Geometry check sheet. Reference: the model listing, model coordinates, mm. Face numbers are marked on the shaded views. Coordinates: 2 decimals unless noted, no trailing zeros. Write each loop counter-clockwise with the first axis right and the second up, starting at its lowest first coordinate (ties: lowest second). Pieces come first, ordered by that corner, then holes. Notation, with made-up numbers: (-10.75, -16.5) -> (4.25, -16.5) arc R27 cw to (4.25, 2.5) -> close; hole circle Ø3 at (4, 9.25). An arc over 180 degrees is marked (long way). Answer in a Markdown table with one row per item. Add a question column.
1. Mould release check, pull along Z, two halves, no side actions. Record for the marked faces 1, 2, 3 and 4: pulls with the +Z half, pulls with the -Z half, needs draft (parallel to the pull), parting line crosses it, or undercut.
2. Scan lines: L1, parallel to Z at x = 1303.5, y = 13.5; L2, parallel to Z at x = 1605, y = 19; L3, parallel to X at y = 12, z = -637. Record each from-to range of solid material in increasing order. Write a range as from..to.
3. Cross-section at B-B on x = 790. Record the cut outline in (y, z).
4. Depth check by flat-ended pin: P1, Ø1, axis at y = 34.5, z = -697.5, coming from the +X side. Enter the tip coordinate at first touch or a pass-through.
5. Cross-section at A-A on z = -89. Record the cut outline in (x, y).
6. Cross-section at C-C on y = 68. Record the cut outline in (x, z).
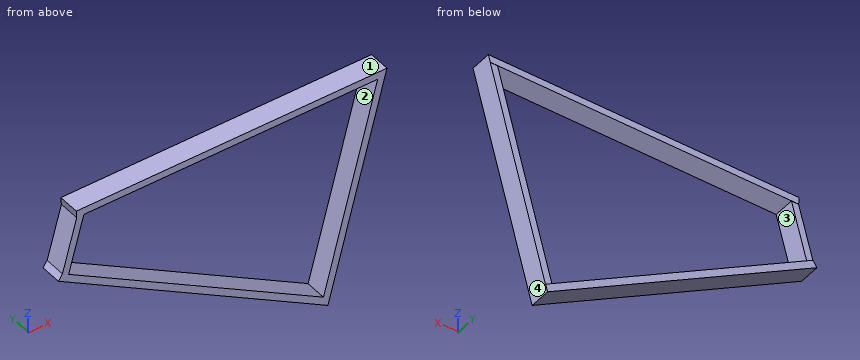
Autodesk Inventor part; units mm, degrees
ref_plane "YZ Plane" through (0, 0, 0) normal (1, 0, 0) x (0, 1, 0)
ref_plane "XZ Plane" through (0, 0, 0) normal (0, 1, 0) x (-1, 0, 0)
ref_plane "XY Plane" through (0, 0, 0) normal (0, 0, 1) x (1, 0, 0)
sketch "Sketch1" plane through (0, 0, 0) normal (0, 1, 0) x (-1, 0, 0)
  line L0 (0, 0) -> (-3000, 0) construction
  line L1 (0, 0) -> (-2598.0762, -1500) construction
  line L2 (0, 0) -> (3000, 0) construction
  arc A0 (-497.4937, 50) -> (-402.0602, -297.2332) centre (0, 0) ccw
  line L3 (-497.4937, 50) -> (-2157.4937, 50)
  line L4 (-2157.4937, 50) -> (-1841.7345, -1128.4295)
  line L5 (-2157.4937, 50) -> (-937.4937, 50) construction
  line L6 (-1841.7345, -1128.4295) -> (1158.2655, -1128.4295) construction
  line L7 (-1841.7345, -1128.4295) -> (-402.0602, -297.2332)
  arc A1 (-537.8662, 12) -> (-456.459, -284.7617) centre (0, 0) ccw
  line L8 (-2107.9712, 12) -> (-537.8662, 12)
  line L9 (-456.459, -284.7617) -> (-1817.8467, -1070.7593)
  line L10 (-2107.9712, 12) -> (-1817.8467, -1070.7593)
  dimension "d1" = 3000
  dimension "d2" = 150
  dimension "d3" = 1000
  dimension "d11" = 50
  dimension "d12" = 1660
  dimension "d13" = 1220
  dimension "d14" = 75
extrude "Extrusion2" add sketch "Sketch1" along normal blind 114
sketch "Sketch2" plane through (0, 114, 0) normal (0, 1, 0) x (1, 0, 0)
  line L0 (497.4937, -50) -> (2157.4937, -50)
  line L1 (1841.7345, 1128.4295) -> (402.0602, 297.2332)
  arc A0 (497.4937, -50) -> (402.0602, 297.2332) centre (0, 0) ccw
  line L2 (456.459, 284.7617) -> (537.8662, -12)
  line L3 (456.459, 284.7617) -> (423.5293, 265.7497)
  line L4 (537.8662, -12) -> (499.856, -12)
  line L5 (423.5293, 265.7497) -> (499.856, -12)
extrude "Extrusion3" add sketch "Sketch2" against normal blind 114 contours L5 A0
sketch "Sketch3" plane through (0, 114, 0) normal (0, 1, 0) x (1, 0, 0)
  arc A0 (537.8662, -12) -> (456.459, 284.7617) centre (0, 0) ccw
  line L0 (456.459, 284.7617) -> (537.8662, -12)
extrude "Extrusion4" cut sketch "Sketch3" against normal blind 3500
sketch "Sketch4" plane through (0, 114, 0) normal (0, 1, 0) x (1, 0, 0)
  line L0 (537.8662, -12) -> (456.459, 284.7617)
  line L1 (2107.9712, -12) -> (537.8662, -12)
  line L2 (1841.7345, 1128.4295) -> (402.0602, 297.2332)
  line L3 (423.5293, 265.7497) -> (499.856, -12)
  line L4 (456.459, 284.7617) -> (423.5293, 265.7497)
  line L5 (499.856, -12) -> (537.8662, -12)
extrude "Extrusion5" cut sketch "Sketch4" against normal blind 1
sketch "Sketch5" plane through (0, 114, 0) normal (0, 1, 0) x (1, 0, 0)
  line L0 (1817.8467, 1070.7593) -> (2107.9712, -12)
  line L1 (497.4937, -50) -> (2157.4937, -50)
  line L2 (2157.4937, -50) -> (1841.7345, 1128.4295)
  line L3 (1841.7345, 1128.4295) -> (402.0602, 297.2332)
  line L4 (1817.8467, 1070.7593) -> (1851.9166, 1090.4295)
  line L5 (2107.9712, -12) -> (2147.3116, -12)
extrude "Extrusion6" cut sketch "Sketch5" against normal blind 1
properties part number "panelAflat" material "Wood (Birch)"
Results found:
| question | item | result |
|---|---|---|
| 1 | face 1 | pulls with the +Z half |
| 1 | face 2 | undercut |
| 1 | face 3 | undercut |
| 1 | face 4 | pulls with the -Z half |
| 2 | L1 | z = -817.68..-773.8, 12..50 |
| 2 | L2 | z = -991.75..-947.87, 12..50 |
| 2 | L3 | x = 990.55..1066.55, 1934.07..1973.41 |
| 3 | outline | (0, -521.21) -> (114, -521.21) -> (114, -477.33) -> (0, -477.33) -> close; (0, 12) -> (114, 12) -> (114, 50) -> (0, 50) -> close |
| 4 | P1 | stops at x = 1957.34 |
| 5 | outline | (472.1, 0) -> (510.16, 0) -> (510.16, 113) -> (472.1, 113) -> close; (2080.91, 0) -> (2120.25, 0) -> (2120.25, 113) -> (2080.91, 113) -> close |
| 6 | outline | (402.06, -297.23) -> (1841.73, -1128.43) -> (2157.49, 50) -> (497.49, 50) arc R500 cw to (499.86, 12) -> (423.53, -265.75) arc R500 cw to start; hole (456.46, -284.76) -> (1817.85, -1070.76) -> (2107.97, 12) -> (537.87, 12) -> close |
